Autodesk Inventor part; units mm, degrees
ref_plane "YZ Plane" through (0, 0, 0) normal (1, 0, 0) x (0, 1, 0)
ref_plane "XZ Plane" through (0, 0, 0) normal (0, 1, 0) x (-1, 0, 0)
ref_plane "XY Plane" through (0, 0, 0) normal (0, 0, 1) x (1, 0, 0)
sketch "Sketch1" plane through (0, 0, 0) normal (0, 1, 0) x (-1, 0, 0)
  line L0 (-5, 16) -> (5, 16)
  line L1 (5, 16) -> (5, -16)
  line L2 (5, -16) -> (-5, -16)
  line L3 (-5, -16) -> (-5, 16)
  line L4 (-5, 16) -> (5, -16) construction
  line L5 (5, 16) -> (-5, -16) construction
  point P0 (0, 0)
  dimension "d0" = 32
  dimension "d1" = 10
extrude "Extrusion1" add sketch "Sketch1" along normal blind 10
sketch "Sketch2" plane through (0, 10, 0) normal (0, 1, 0) x (1, 0, 0)
  line L0 (0, 22.4) -> (0, -22.4)
  line L1 (7, 0) -> (-7, 0)
  point P0 (0, 0)
  point P1 (0, -11)
  point P2 (0, 11)
  dimension "d4" = 22
hole "Hole1" at (0, 10, 11) at (0, 10, -11) direction (0, -1, 0) diameter 3.4 depth 10 counterbore diameter 6.5 counterbore depth 3.4
fillet "Fillet1" radius 2 4 edges at (5, 5, 16) (-5, 5, 16) (5, 5, -16) (-5, 5, -16)
sketch "Sketch3" plane through (5, 0, 14) normal (1, 0, 0) x (0, 0, -1)
  line L0 (28, 0) -> (0, 0)
  line L1 (6.5, 0) -> (21.5, 0)
  line L2 (21.5, 0) -> (21.5, 2)
  line L3 (21.5, 2) -> (6.5, 2)
  line L4 (6.5, 2) -> (6.5, 0)
  line L5 (14, -2) -> (14, 12)
  point P0 (14, 0)
  dimension "d13" = 15
  dimension "d14" = 2
extrude "Extrusion2" cut sketch "Sketch3" against normal through all
fillet "Fillet2" radius 2 4 edges at (5, 1, 7.5) (-5, 1, 7.5) (5, 1, -7.5) (-5, 1, -7.5)
properties part number "32_Y-Motor_cable_holder_B"
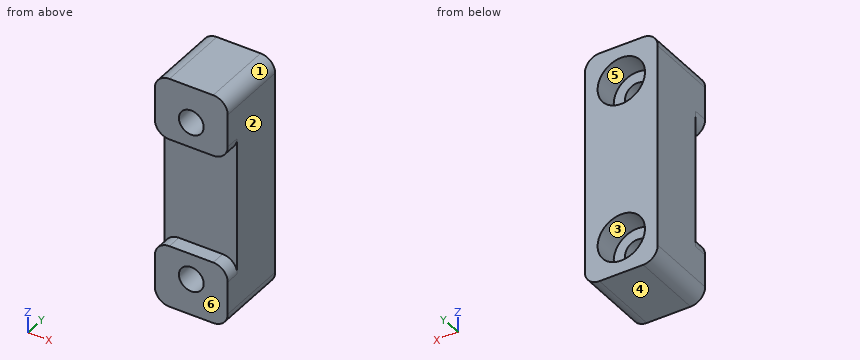
Build history of the part. All positions in model axes, mm. Face numbers are marked on the shaded views. A direction names the side the tool comes from. Give positions to 0.01 mm unless a question says otherwise; leave off trailing zeros. Loops run counter-clockwise (first coordinate to the right, second up) from the corner with the lowest first, then second, coordinate; pieces in that order, holes last. Notation, with made-up numbers: (-30.5, 36) - (14.5, 36) arc R10 ccw to (14.5, 50) - close; hole circle Ø8 at (48.5, 60.5). An arc over 180 degrees is marked (long way). Write item = value, one per line. Start each with the question number.
1) Drop flat-ended pins along their axis: pin 1 Ø1 at (x, z) = (0, 0) entering from -Y; pin 2 Ø5 at (x, z) = (0.5, 11.5) entering from +Y. Give the stop position or say it passes through.
2) Probe probe 1 along Z at (x, y) = (0, 2.75); probe 2 along Z at (x, y) = (0, 7.8); probe 3 along X at (y, z) = (4.25, -11). List the from-to ranges inside material, lowest first. Write a range as from..to.
3) Band-saw the part on D-D on x = 1.25. Give the cut face in (y, z).
4) Tool access for the marked faces 5 and 6: list every direction of +Z, -Z, +X, -X, +Y, -Y with a clear straight run to the whole face (end or side of a thin tool).
5) Pull direction Z, two halves, no side cores. Call the marked faces 1, 2, 3 and 4: +Z half, -Z half, draft (parallel to the pull), parting line (faces both ways), or undercut.
6) Band-saw the part on C-C on y = 8.25. Give the cut face in (x, z).
7) Band-saw the part on A-A on x = 0. Give the cut face in (y, z), plus the area to 3 significant figures.
8) Band-saw the part on B-B on z = -11. Give the cut face in (x, y).
Final values:
q1.pin_1 = 2
q1.pin_2 = 6.6
q2.probe_1 = -16..-12.7, -9.3..9.3, 12.7..16
q2.probe_2 = -16..-14.25, -7.75..7.75, 14.25..16
q2.probe_3 = -5..-1.7, 1.7..5
q3.outline = (0, -16) - (10, -16) - (10, -14) - (6.6, -14) - (6.6, -12.15) - (0, -12.15) - close; (0, -9.85) - (6.6, -9.85) - (6.6, -8) - (10, -8) - (10, 8) - (6.6, 8) - (6.6, 9.85) - (0, 9.85) - (0, 7.5) - (2, 7.5) - (2, -7.5) - (0, -7.5) - close; (0, 12.15) - (6.6, 12.15) - (6.6, 14) - (10, 14) - (10, 16) - (0, 16) - close
q4.face_5 = +Y
q4.face_6 = +Z, -Z, +X, -X, -Y
q5.face_1 = +Z half
q5.face_2 = draft
q5.face_3 = undercut
q5.face_4 = -Z half
q6.outline = (-5, -14) arc R2 ccw to (-3, -16) - (3, -16) arc R2 ccw to (5, -14) - (5, 14) arc R2 ccw to (3, 16) - (-3, 16) arc R2 ccw to (-5, 14) - close; hole circle Ø6.5 at (0, -11); hole circle Ø6.5 at (0, 11)
q7.outline = (0, -16) - (10, -16) - (10, -14.25) - (6.6, -14.25) - (6.6, -12.7) - (0, -12.7) - close; (0, -9.3) - (6.6, -9.3) - (6.6, -7.75) - (10, -7.75) - (10, 7.75) - (6.6, 7.75) - (6.6, 9.3) - (0, 9.3) - (0, 7.5) - (2, 7.5) - (2, -7.5) - (0, -7.5) - close; (0, 12.7) - (6.6, 12.7) - (6.6, 14.25) - (10, 14.25) - (10, 16) - (0, 16) - close
q7.area = 201 mm²
q8.outline = (-5, 0) - (-1.7, 0) - (-1.7, 6.6) - (-3.25, 6.6) - (-3.25, 10) - (-5, 10) - close; (1.7, 0) - (5, 0) - (5, 10) - (3.25, 10) - (3.25, 6.6) - (1.7, 6.6) - close
